Can you work these out from the drawing? Everything is in mm from the part's minimum corner. A direction names the side the tool comes from. Round coordinates to 2 decimals unless told otherwise and drop trailing zeros. Write each loop counter-clockwise with the first axis right and the second up, starting at its lowest first coordinate (ties: lowest second). Pieces come first, ordered by that corner, then holes. Notation, with made-up numbers: (46.5, 69) - (59.5, 69) arc R19 cw to (59.5, 97) - close; hole circle Ø11 at (-4, 18.25). An arc over 180 degrees is marked (long way). Write each question's results on one line, items separated by ' | '. Start each with the question number.
(1) Imagine slicing it at A-A on x = 34. Write out the boundary of the cut face in (y, z) (1 decimal), then the cut area to 3 significant figures.
(2) Imagine slicing it at D-D on y = 25.5. Write out the boundary of the cut face in (x, z).
(3) Imagine slicing it at C-C on y = 66.5. Write out the boundary of the cut face in (x, z).
(4) On a 3-axis mill with a long thin cutter (end or side, diameter ignored), from which of +Z, -Z, +X, -X, +Y, -Y can I reach the whole of each face in a straight line? I mean the marked faces 1, 2 and 3. Say none if no direction works.
(5) For P1, Ø3.5, axis at x = 58, z = 51.5, coming from the -Y side; P2, Ø18.5, axis at x = 29.5, y = 62, coming from the +Z side; P3, Ø1, axis at x = 18.5, z = 9.5, coming from the +Y side, each with a flat end and sliding along its axis, tell me the tip position at first contact or that it passes through.
(6) Please list where these lines run through material, in increasing order: line 1 (Y direction, x = 10, z = 11.5); line 2 (Z direction, x = 15.5, y = 11.5); line 3 (X direction, y = 13.5, z = 26). Write a range as [from, to].
(7) Imagine slicing it at B-B on z = 40. Write out the boundary of the cut face in (x, y) (1 decimal).
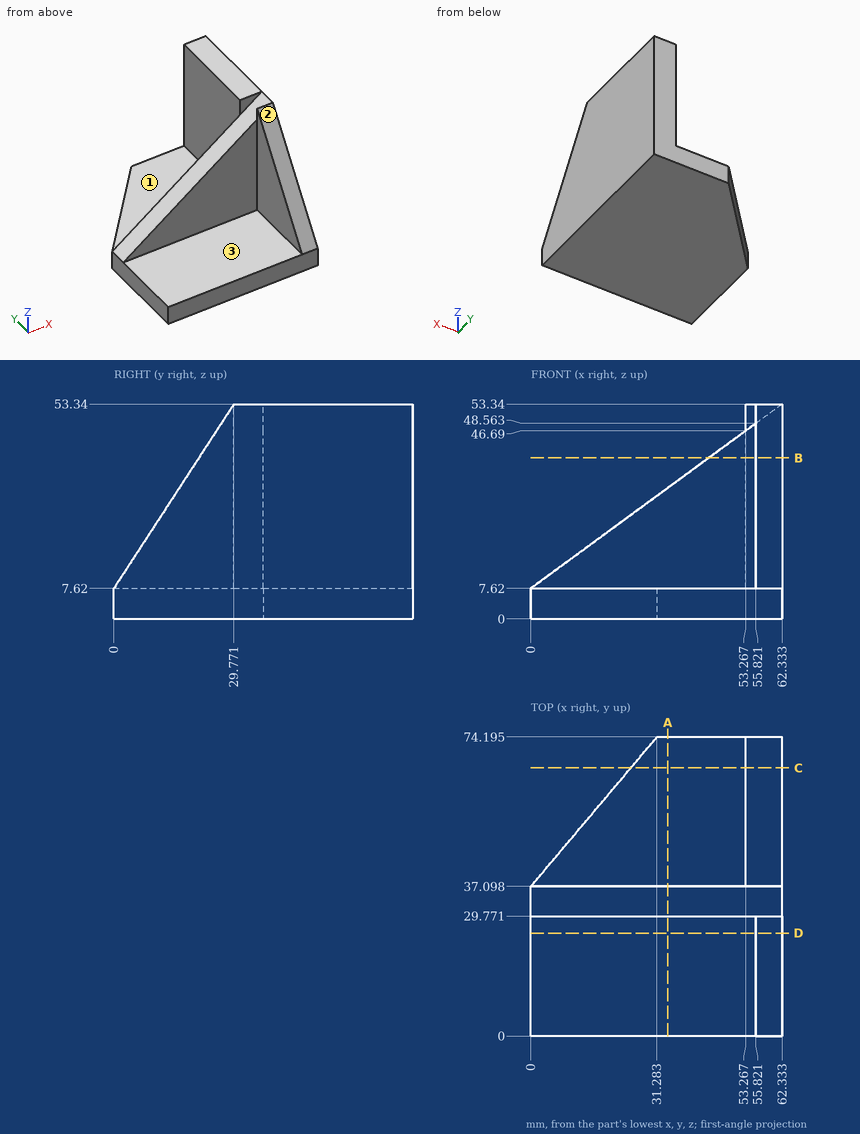
Response:
1) outline: (0, 0) - (74.2, 0) - (74.2, 7.6) - (37.1, 7.6) - (37.1, 32.6) - (29.8, 32.6) - (29.8, 7.6) - (0, 7.6) - close | area: 748 mm²
2) outline: (0, 0) - (62.33, 0) - (62.33, 46.78) - (55.82, 46.78) - (55.82, 7.62) - (0, 7.62) - close
3) outline: (24.79, 0) - (62.33, 0) - (62.33, 53.34) - (53.27, 53.34) - (53.27, 7.62) - (24.79, 7.62) - close
4) face 1: +Z, -X, +Y | face 2: +Z, +X, -X, -Y | face 3: +Z, -X, -Y
5) P1: y = 27.43 | P2: z = 7.62 | P3: y = 37.1
6) line 1: [29.77, 37.1] | line 2: [0, 7.62] | line 3: [55.82, 62.33]
7) outline: (44.1, 29.8) - (55.8, 29.8) - (55.8, 21.1) - (62.3, 21.1) - (62.3, 74.2) - (53.3, 74.2) - (53.3, 37.1) - (44.1, 37.1) - close
